Could you check a few things on this model? Use its own coordinates, in mm. Face numbers are marked on the shaded views. A direction names the side the tool comes from. Coordinates: 2 decimals unless noted, no trailing zeros. Write each loop counter-clockwise with the first axis right and the second up, starting at its lowest first coordinate (ties: lowest second). Pieces come first, ordered by that corner, then holes. Notation, with made-up numbers: M 11,84.25 L 37,84.25 A23 cw 37,109.25 Z; hole C -0.5,74.25 d1. An arc over 180 degrees is marked long. Write item = value, one per line.
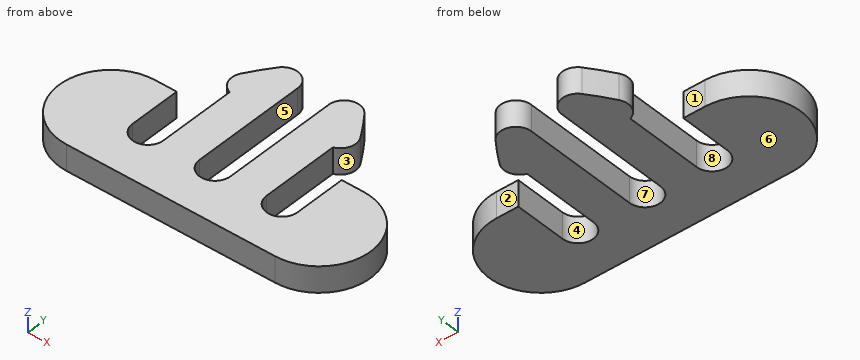
```python
from build123d import *

# Parameters (mm, degrees)
BOSS_EXTRUDE1_DEPTH = 2.5
CUT_EXTRUDE1_START  = -2.5
CUT_EXTRUDE1_DEPTH  = 2.5
FILLET1_R           = 1.5
FILLET2_R           = 1.5


with BuildPart() as part:
    # Sketch1 → Boss-Extrude1 (new body)
    with BuildSketch(Plane.XY):
        with BuildLine():
            Line((-22.837615564, 46.083177434), (-27.937615564, 46.083177434))
            ThreePointArc((-27.937615564, 46.083177434), (-32.937615564, 41.083177434), (-27.937615564, 36.083177434))
            Line((-27.937615564, 36.083177434), (-7.737615564, 36.083177434))
            ThreePointArc((-7.737615564, 36.083177434), (-2.737615564, 41.083177434), (-7.737615564, 46.083177434))
            Line((-7.737615564, 46.083177434), (-12.837615564, 46.083177434))
            Line((-12.837615564, 46.083177434), (-12.837615564, 48.583177434))
            Line((-12.837615564, 48.583177434), (-10.837615564, 48.583177434))
            add(Edge.make_bspline(
                [(-16.337615564, 56.083177434), (-12.915611401, 52.825980487), (-10.837615564, 48.583177434)],
                knots=[0, 0, 0, 1, 1, 1], degree=2))
            Line((-16.337615564, 56.083177434), (-16.337615564, 46.083177434))
            ThreePointArc((-16.337615564, 46.083177434), (-17.837615564, 44.583177434), (-19.337615564, 46.083177434))
            Line((-19.337615564, 46.083177434), (-19.337615564, 56.083177434))
            add(Edge.make_bspline(
                [(-19.337615564, 56.083177434), (-22.759619727, 52.825980487), (-24.837615564, 48.583177434)],
                knots=[0, 0, 0, 1, 1, 1], degree=2))
            Line((-24.837615564, 48.583177434), (-22.837615564, 48.583177434))
            Line((-22.837615564, 48.583177434), (-22.837615564, 46.083177434))
        make_face()
    extrude(amount=BOSS_EXTRUDE1_DEPTH)

    # Sketch2 → Cut-Extrude1 (cut)
    with BuildSketch(Plane.XY.offset(2.5).offset(CUT_EXTRUDE1_START)):
        with BuildLine():
            Line((-9.837615564, 46.083177434), (-9.837615564, 41.083177434))
            ThreePointArc((-9.837615564, 41.083177434), (-11.337615564, 39.583177434), (-12.837615564, 41.083177434))
            Line((-12.837615564, 41.083177434), (-12.837615564, 46.083177434))
            ThreePointArc((-12.837615564, 46.083177434), (-11.337615564, 47.583177434), (-9.837615564, 46.083177434))
        make_face()
        with BuildLine():
            Line((-25.837615564, 46.083177434), (-25.837615564, 41.083177434))
            ThreePointArc((-25.837615564, 41.083177434), (-24.337615564, 39.583177434), (-22.837615564, 41.083177434))
            Line((-22.837615564, 41.083177434), (-22.837615564, 46.083177434))
            ThreePointArc((-22.837615564, 46.083177434), (-24.337615564, 47.583177434), (-25.837615564, 46.083177434))
        make_face()
        with BuildLine():
            Line((-19.337615564, 46.083177434), (-19.337615564, 41.083177434))
            ThreePointArc((-19.337615564, 41.083177434), (-17.837615564, 39.583177434), (-16.337615564, 41.083177434))
            Line((-16.337615564, 41.083177434), (-16.337615564, 46.083177434))
            ThreePointArc((-16.337615564, 46.083177434), (-17.837615564, 47.583177434), (-19.337615564, 46.083177434))
        make_face()
    extrude(amount=CUT_EXTRUDE1_DEPTH, mode=Mode.SUBTRACT)

    # Fillet1
    # the kernel refuses this fillet: 1.5 mm, written as the material it takes off along each edge
    with BuildSketch(Plane(origin=(-10.837615564, 48.583177434, -6.280550784), x_dir=(-1, 0, 0), z_dir=(0, 0, 1))) as fillet1_piece_1:
        with BuildLine():
            CenterArc((2.488462024, -1.418240054), FILLET1_R, 109.004435481, 102.492563124)
            Line((1.209460724, -2.201920903), (1.183880698, -2.21759452))
            ThreePointArc((1.183880698, -2.21759452), (0.552459457, -1.12966162), (-0.026942162, -0.013195451))
            Line((-0.026942162, -0.013195451), (0, 0.03))
            ThreePointArc((0, 0.03), (1, 0.03), (1.99023076, 0.028364801))
            Line((1.99023076, 0.028364801), (2, 0))
        make_face()
    extrude(amount=15.061101567, mode=Mode.SUBTRACT)
    with BuildSketch(Plane(origin=(-24.837615564, 48.583177434, -6.280550784), x_dir=(1, 0, 0), z_dir=(0, 0, 1))) as fillet1_piece_2:
        with BuildLine():
            CenterArc((2.488462024, 1.418240054), FILLET1_R, 148.503001395, 102.492563124)
            Line((1.209460724, 2.201920903), (1.183880698, 2.21759452))
            ThreePointArc((1.183880698, 2.21759452), (0.552459457, 1.12966162), (-0.026942162, 0.013195451))
            Line((-0.026942162, 0.013195451), (0, -0.03))
            ThreePointArc((0, -0.03), (1, -0.03), (1.99023076, -0.028364801))
            Line((1.99023076, -0.028364801), (2, 0))
        make_face()
    extrude(amount=15.061101567, mode=Mode.SUBTRACT)

    # Fillet2
    fillet2_edges = [part.edges().sort_by_distance(p)[0] for p in [
        (-16.337615564, 56.083177434, 1.25),
        (-19.337615564, 56.083177434, 1.25),
    ]]
    fillet(fillet2_edges, radius=FILLET2_R)


solid = part.part
```
Item 1: Imagine slicing it at A-A (y = 47.5). Write out the boundary of the cut face in (x, z), and give its area (3 significant figures).
Numbers:
outline = M -22.84,0 L -19.34,0 L -19.34,2.5 L -22.84,2.5 Z; M -16.34,0 L -12.84,0 L -12.84,2.5 L -16.34,2.5 Z
area = 17.5 mm²
Item 2: If I drill on line 1 along X through (y, z) = (41.25, 1.75); line 2 along X through (y, z) = (47.75, 0.4); line 3 along X through (y, z) = (42, 0.8), over which ranges is the centre line in solid material (lowest first)?
Numbers:
line_1 = -32.93 to -25.84, -22.84 to -19.34, -16.34 to -12.84, -9.84 to -2.74
line_2 = -22.84 to -19.34, -16.34 to -12.84
line_3 = -32.85 to -25.84, -22.84 to -19.34, -16.34 to -12.84, -9.84 to -2.82
Item 3: For the marked faces 1, 2, 3, 4 and 5, which set-ups out of +Z, -Z, +X, -X, +Y, -Y let a thin tool reach every point of the face, with its end or its side?
Numbers:
face_1 = +Z, -Z, -X, +Y
face_2 = +Z, -Z, +X, +Y
face_3 = +Z, -Z, +X
face_4 = +Z, -Z
face_5 = +Z, -Z, +Y
Item 4: Imagine slicing it at B-B (y = 43.25). Write out the boundary of the cut face in (x, z).
Numbers:
outline = M -32.44,0 L -25.84,0 L -25.84,2.5 L -32.44,2.5 Z; M -22.84,0 L -19.34,0 L -19.34,2.5 L -22.84,2.5 Z; M -16.34,0 L -12.84,0 L -12.84,2.5 L -16.34,2.5 Z; M -9.84,0 L -3.23,0 L -3.23,2.5 L -9.84,2.5 Z
Item 5: I'm going to push flat-ended pins straight in: P1, Ø0.8, axis at y = 44, z = 1.5, coming from the +X side; P2, Ø0.8, axis at y = 45, z = 1, coming from the +X side; P3, Ø0.6, axis at x = -9, z = 0.5, coming from the +Y side. Where does each tip first touch, or does it pass through?
Numbers:
P1 = -3.42
P2 = -4.18
P3 = 46.08
Item 6: If we mould it in two halves opening along Y, with no side actions, what happens to the marked faces 6, 7 and 8? For each: pulls with the +Y half, pulls with the -Y half, needs draft (parallel to the pull), parting line crosses it, or undercut.
Numbers:
face_6 = needs draft
face_7 = pulls with the +Y half
face_8 = undercut
Item 7: Imagine slicing it at C-C (y = 37.75). Write out the boundary of the cut face in (x, z).
Numbers:
outline = M -31.66,0 L -4.01,0 L -4.01,2.5 L -31.66,2.5 Z
